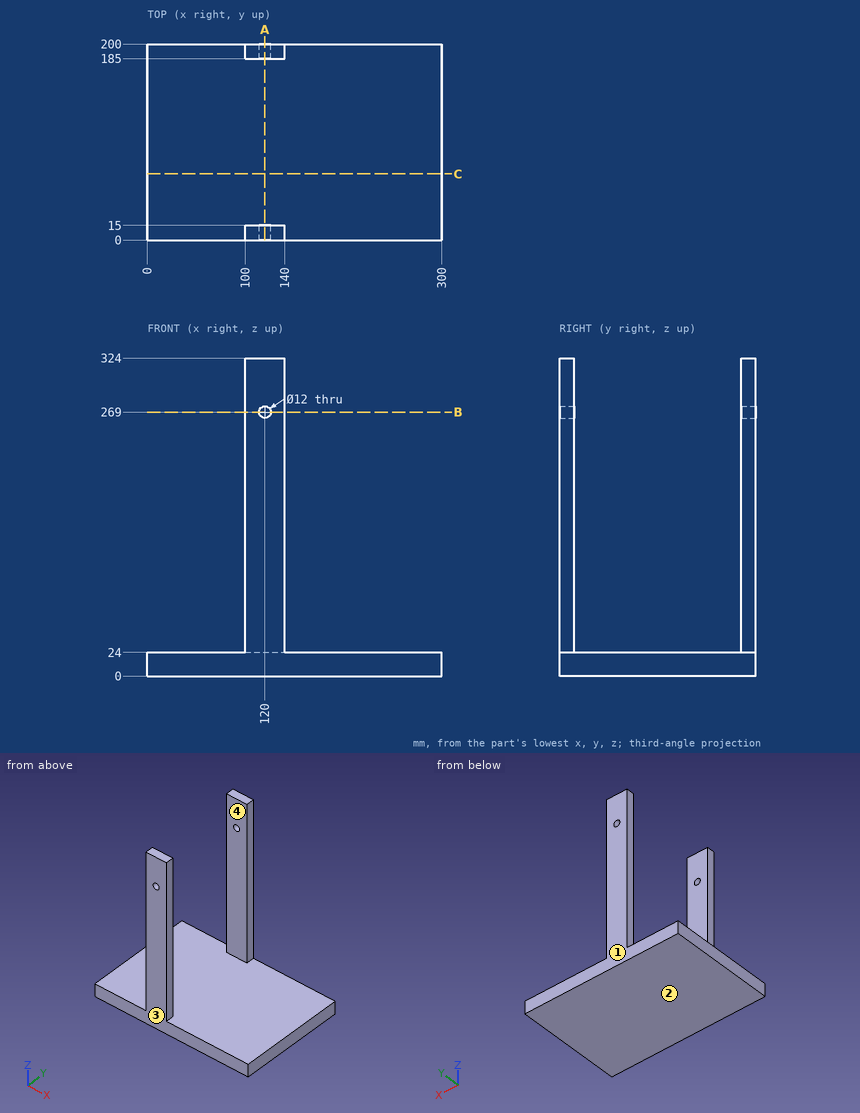
Design review of the part shown in the three views and the two pictorial views. Dimensions are in mm from the part's minimum x, y and z. Round coordinates to 2 decimals unless told otherwise and drop trailing zeros. Order: outer loops, then holes, each group sorted by start corner. A loop starts at its lowest first (then second) coordinate and runs counter-clockwise, first axis right, second up.
Q1. We need section A-A, the plane x = 120. Give the boundary of the cut face in (y, z).
Findings below:
outline: (0, 0) - (200, 0) - (200, 263) - (185, 263) - (185, 24) - (15, 24) - (15, 263) - (0, 263) - close; (0, 275) - (15, 275) - (15, 324) - (0, 324) - close; (185, 275) - (200, 275) - (200, 324) - (185, 324) - close
Q2. Insertion check: P1, Ø4.5, axis at y = 8, z = 135.5, coming from the +X side; P2, Ø7.5, axis at y = 8, z = 174.5, coming from the -X side. Each pin has a flat end and moves straight along its axis. Give the tip position at first contact, or say it passes through.
Findings below:
P1: stops at x = 140
P2: stops at x = 100
Q3. We need section B-B, the plane z = 269. Give the boundary of the cut face in (x, y), plus the area to 3 significant figures.
Findings below:
outline: (100, 0) - (114, 0) - (114, 15) - (100, 15) - close; (100, 185) - (114, 185) - (114, 200) - (100, 200) - close; (126, 0) - (140, 0) - (140, 15) - (126, 15) - close; (126, 185) - (140, 185) - (140, 200) - (126, 200) - close
area: 840 mm2
Q4. Mouldability with a two-part tool opening along Y and no side actions: class the marked faces 1, 2, 3 and 4 as pulls with the +Y half, pulls with the -Y half, needs draft (parallel to the pull), parting line crosses it, or undercut.
Findings below:
face 1: pulls with the +Y half
face 2: needs draft
face 3: pulls with the -Y half
face 4: undercut
Q5. Wall thickness on line 1 (X direction, y = 9.5, z = 269); line 2 (Y direction, x = 100.5, z = 88.5); line 3 (Z direction, x = 120, y = 193.75): over which ranges is each line inside the solid? List them lowest first.
Findings below:
line 1: x = 100 to 114, 126 to 140
line 2: y = 0 to 15, 185 to 200
line 3: z = 0 to 263, 275 to 324
Q6. We need section C-C, the plane y = 67.5. Give the boundary of the cut face in (x, z), plus the area to 3 significant figures.
Findings below:
outline: (0, 0) - (300, 0) - (300, 24) - (0, 24) - close
area: 7,200 mm2
